Check sheet for the modelled part. Datum: model origin and axes. Units: mm. Give positions to 0.01 mm unless a question says otherwise; leave off trailing zeros. Loops run counter-clockwise (first coordinate to the right, second up) from the corner with the lowest first, then second, coordinate; pieces in that order, holes last. Notation, with made-up numbers: (-28.5, 44.5) -> (-17.5, 44.5) arc R13 cw to (-17.5, 54.5) -> close; hole circle Ø11 at (-40, 60). An arc over 180 degrees is marked (long way). Answer as CSV lines item,"result". Start each with the question number.
(1) Gauge pin test, flat end, axial feed: pin 1 Ø1.2 at (x, y) = (0, 0) entering from +Z. Record the tip position at first contact, or that the pin passes through.
(2) Section check A-A on x = 0. Enter the section's corners in (y, z).
(3) Section check C-C on z = 3.75. Enter the section's corners in (x, y).
(4) Release check for a two-part mould opening along X. For faces 1 (the face through (-0.27, -1.22, 5.92)), 2 (the face through (-0.54, -2.44, 7.2)), 3 (the face through (0, -1, 13)), 4 (the face through (-1, -1, 15)) record: pulls with the +X half, pulls with the -X half, needs draft (parallel to the pull), parting line crosses it, or undercut.
(5) Material ranges on line 1 (Y direction, x = 0, z = 3); line 2 (Y direction, x = 0, z = 12.5); line 3 (X direction, y = -0.4, z = 9.25), recorded low to high. Write a range as from..to.
from build123d import *

# Parameters (mm, degrees)
SKETCH1_R                       = 2.5
BOSS_EXTRUDE1_DEPTH             = 15
SKETCH2_R                       = 1
CUT_EXTRUDE1_DEPTH              = 16
TAP_DRILL_FOR_M3X0_5_TAP1_D     = 2.5
TAP_DRILL_FOR_M3X0_5_TAP1_DEPTH = 11
TAP_DRILL_FOR_M3X0_5_TAP1_TIP   = 0.751075774
CHAMFER1_SIZE                   = 0.4
CHAMFER1_SIZE2                  = 0.230940108
CHAMFER2_SIZE                   = 0.4
CHAMFER2_SIZE2                  = 0.692820323


with BuildPart() as part:
    # Sketch1 → Boss-Extrude1 (new body)
    with BuildSketch(Plane.XY):
        Circle(SKETCH1_R)
    extrude(amount=BOSS_EXTRUDE1_DEPTH)

    # Sketch2 → Cut-Extrude1 (cut, through all)
    with BuildSketch(Plane(origin=(0, 0, 0), x_dir=(-1, 0, 0), z_dir=(0, 0, -1))):
        Circle(SKETCH2_R)
    extrude(amount=-CUT_EXTRUDE1_DEPTH, mode=Mode.SUBTRACT)

    # Tap Drill for M3x0.5 Tap1
    with Locations(Plane(origin=(0, 0, 0), x_dir=(-1, 0, 0), z_dir=(0, 0, -1))):
        with Locations((0, 0)):
            Hole(TAP_DRILL_FOR_M3X0_5_TAP1_D / 2, depth=TAP_DRILL_FOR_M3X0_5_TAP1_DEPTH)
            with Locations((0, 0, -(TAP_DRILL_FOR_M3X0_5_TAP1_DEPTH + TAP_DRILL_FOR_M3X0_5_TAP1_TIP / 2))):  # 118° drill point
                Cone(0, TAP_DRILL_FOR_M3X0_5_TAP1_D / 2, TAP_DRILL_FOR_M3X0_5_TAP1_TIP, mode=Mode.SUBTRACT)

    # Chamfer1
    chamfer1_edges = [part.edges().sort_by_distance(p)[0] for p in [
        (-2.5, 0, 15),
    ]]
    chamfer1_side = [part.faces().sort_by_distance(p)[0] for p in [
        (-2.5, 0, 7.5),
    ]]
    chamfer(chamfer1_edges, length=CHAMFER1_SIZE, length2=CHAMFER1_SIZE2, reference=chamfer1_side[0])

    # Chamfer2
    chamfer2_edges = [part.edges().sort_by_distance(p)[0] for p in [
        (-1.25, 0, 0),
    ]]
    chamfer2_side = [part.faces().sort_by_distance(p)[0] for p in [
        (-2.429289322, 0, 0),
    ]]
    chamfer(chamfer2_edges, length=CHAMFER2_SIZE, length2=CHAMFER2_SIZE2, reference=chamfer2_side[0])


solid = part.part
Working result:
1,pin 1,"passes through"
2,outline,"(-2.5, 0) -> (-1.65, 0) -> (-1.25, 0.69) -> (-1.25, 11) -> (-1, 11.15) -> (-1, 15) -> (-2.27, 15) -> (-2.5, 14.6) -> close; (1, 11.15) -> (1.25, 11) -> (1.25, 0.69) -> (1.65, 0) -> (2.5, 0) -> (2.5, 14.6) -> (2.27, 15) -> (1, 15) -> close"
3,outline,"circle Ø5 at (0, 0); hole circle Ø2.5 at (0, 0)"
4,face 1,"undercut"
4,face 2,"parting line crosses it"
4,face 3,"undercut"
4,face 4,"needs draft"
5,line 1,"y = -2.5..-1.25, 1.25..2.5"
5,line 2,"y = -2.5..-1, 1..2.5"
5,line 3,"x = -2.47..-1.18, 1.18..2.47"
